Can you work these out from the drawing? Everything is in mm from the part's minimum corner. A direction names the side the tool comes from. Coordinates: 2 decimals unless noted, no trailing zeros. Write each loop counter-clockwise with the first axis right and the second up, starting at its lowest first coordinate (ties: lowest second). Pieces come first, ordered by that corner, then holes. Notation, with made-up numbers: (67, 46.25) -> (98, 46.25) arc R26 ccw to (98, 73.25) -> close; hole circle Ø8 at (48.5, 76). An arc over 180 degrees is marked (long way). Use a Markdown table: item, result. Add a question column.
Item 1: Imagine slicing it at C-C, the plane y = 12.5. Write out the boundary of the cut face in (x, z), and give its area (3 significant figures).
Item 2: Imagine slicing it at A-A, the plane y = 53. Write out the boundary of the cut face in (x, z) (1 decimal), and give its area (3 significant figures).
Item 3: If we mould it in two halves opening along X, with no side actions, what happens to the marked faces 1, 2 and 3? For each: pulls with the +X half, pulls with the -X half, needs draft (parallel to the pull), parting line crosses it, or undercut.
Item 4: Will these pins go through, and if not, where does the flat tip stop? pin 1 Ø5 at (x, y) = (19.5, 49) entering from -Z; pin 2 Ø1.5 at (x, z) = (24.5, 30) entering from +Y; pin 3 Ø4 at (x, z) = (21.5, 15.5) entering from +Y; pin 4 Ø10 at (y, z) = (36, 34) entering from +X.
Item 5: If I drill on line 1 along X through (y, z) = (27.5, 39.5); line 2 along Y through (x, z) = (27, 37); line 3 along Z through (x, y) = (17.5, 18.5), over which ranges is the centre line in solid material (lowest first)? Write a range as from..to.
Item 6: Imagine slicing it at D-D, the plane x = 25. Write out the boundary of the cut face in (y, z).
Item 7: Imagine slicing it at B-B, the plane z = 39. Write out the boundary of the cut face in (x, y) (1 decimal).
Item 8: On a 3-axis mill with a long thin cutter (end or side, diameter ignored), from which of +Z, -Z, +X, -X, +Y, -Y can I reach the whole of each face in a straight line? I mean the marked faces 4, 5 and 6. Say none if no direction works.
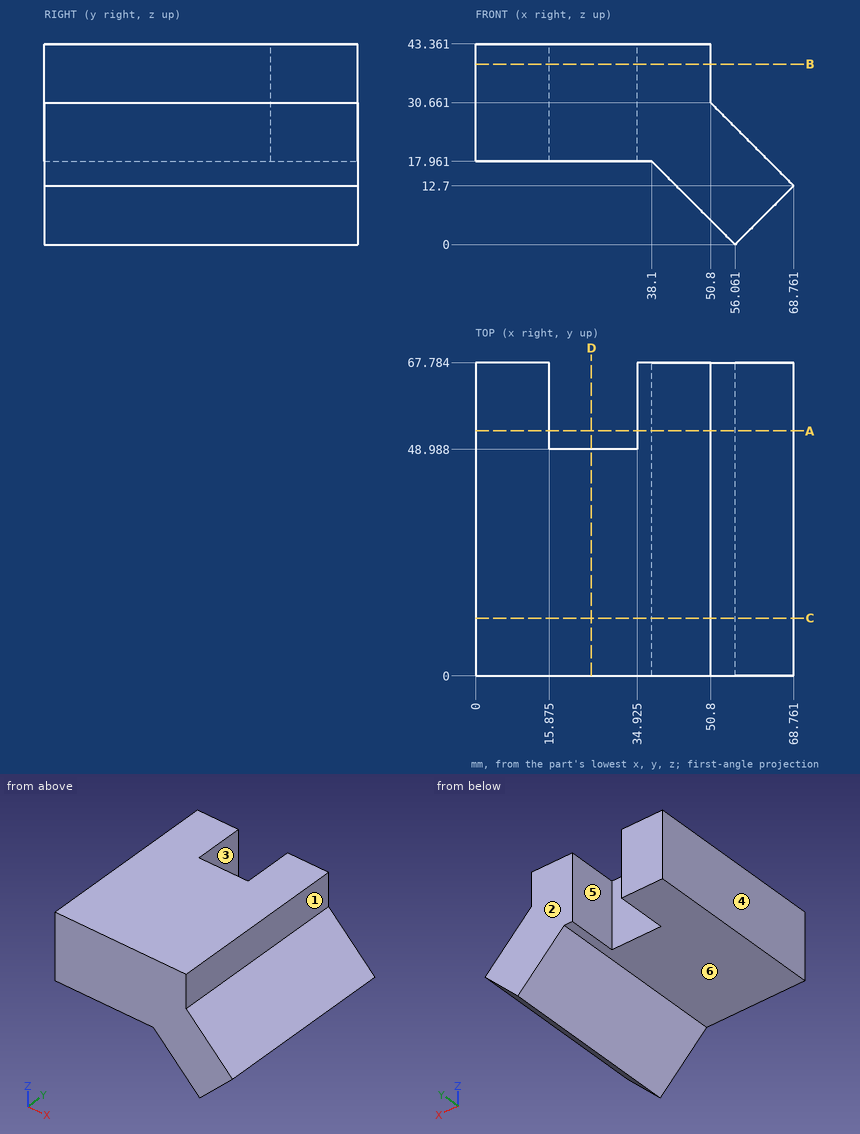
Ans:
| question | item | result |
|---|---|---|
| 1 | outline | (0, 17.96) -> (38.1, 17.96) -> (56.06, 0) -> (68.76, 12.7) -> (50.8, 30.66) -> (50.8, 43.36) -> (0, 43.36) -> close |
| 1 | area | 1,670 mm^2 |
| 2 | outline | (0, 18) -> (15.9, 18) -> (15.9, 43.4) -> (0, 43.4) -> close; (34.9, 18) -> (38.1, 18) -> (56.1, 0) -> (68.8, 12.7) -> (50.8, 30.7) -> (50.8, 43.4) -> (34.9, 43.4) -> close |
| 2 | area | 1,180 mm^2 |
| 3 | face 1 | pulls with the +X half |
| 3 | face 2 | needs draft |
| 3 | face 3 | undercut |
| 4 | pin 1 | stops at z = 17.96 |
| 4 | pin 2 | stops at y = 48.99 |
| 4 | pin 3 | passes through |
| 4 | pin 4 | stops at x = 52.46 |
| 5 | line 1 | x = 0..50.8 |
| 5 | line 2 | y = 0..48.99 |
| 5 | line 3 | z = 17.96..43.36 |
| 6 | outline | (0, 17.96) -> (48.99, 17.96) -> (48.99, 43.36) -> (0, 43.36) -> close |
| 7 | outline | (0, 0) -> (50.8, 0) -> (50.8, 67.8) -> (34.9, 67.8) -> (34.9, 49) -> (15.9, 49) -> (15.9, 67.8) -> (0, 67.8) -> close |
| 8 | face 4 | +Z, -Z, -X, +Y, -Y |
| 8 | face 5 | +Z, -Z, +Y |
| 8 | face 6 | -Z, -X, +Y, -Y |
